Geometry check sheet. Reference: the model listing, model coordinates, mm. A direction names the side the tool comes from. Give positions to 0.01 mm unless a question says otherwise; leave off trailing zeros. Loops run counter-clockwise (first coordinate to the right, second up) from the corner with the lowest first, then second, coordinate; pieces in that order, holes last. Notation, with made-up numbers: (-30.5, 66.25) -> (15.5, 66.25) arc R27 cw to (15.5, 90.25) -> close; hole circle Ø5 at (55, 80). An arc over 180 degrees is marked (long way). Write item = value, one per line.
```python
from build123d import *

# Parameters (mm, degrees)
F0_W     = 12.7
F0_H     = 12.3
F1_DEPTH = 6.35
F2_W     = 6.35
F2_H     = 12.3
F3_DEPTH = 20.32
F4_R     = 1.9939
F5_DEPTH = 12.701
F7_DEPTH = 12.301
F9_DEPTH = 12.701


with BuildPart() as f1:
    # F0 (on Top) → F1 (new body)
    with BuildSketch(Plane.XY):
        Rectangle(F0_W, F0_H)
    extrude(amount=F1_DEPTH)

    # F2 (on face) → F3 (join)
    with BuildSketch(Plane.XY.offset(6.35)):
        with Locations((-3.175, 0)):
            Rectangle(F2_W, F2_H)
    extrude(amount=F3_DEPTH)

    # F4 (on face) → F5 (cut, through all)
    with BuildSketch(Plane.YZ.offset(6.35)):
        with Locations((0, 3.175)):
            Circle(F4_R)
    extrude(amount=-F5_DEPTH, mode=Mode.SUBTRACT)

    # F6 (on face) → F7 (cut, through all)
    with BuildSketch(Plane.XZ.offset(6.15)):
        Polygon((0, 20.955), (0, 23.495), (-2.54, 22.225), align=None)
    extrude(amount=-F7_DEPTH, mode=Mode.SUBTRACT)

    # F8 (on face) → F9 (cut, through all)
    with BuildSketch(Plane.YZ.offset(6.35)):
        with BuildLine():
            Line((-6.15, 5.08), (-6.15, 3.557324))
            ThreePointArc((-6.15, 3.557324), (-5.41976, 4.318662), (-6.15, 5.08))
        make_face()
        with BuildLine():
            Line((-6.15, 2.54), (-6.15, 1.017324))
            ThreePointArc((-6.15, 1.017324), (-5.41976, 1.778662), (-6.15, 2.54))
        make_face()
        with BuildLine():
            ThreePointArc((6.15, 2.54), (5.41976, 1.778662), (6.15, 1.017324))
            Line((6.15, 1.017324), (6.15, 2.54))
        make_face()
        with BuildLine():
            ThreePointArc((6.15, 5.08), (5.41976, 4.318662), (6.15, 3.557324))
            Line((6.15, 3.557324), (6.15, 5.08))
        make_face()
    extrude(amount=-F9_DEPTH, mode=Mode.SUBTRACT)


solid = f1.part
```
Item 1: Draft check along Z on faces 4 (the flat face through (3, 0, 6.35)), 5 (the flat face through (-1.25, -0.09, 22.87)), 6 (the cylindrical face through (0.09, 5.42, 1.79)), 7 (the flat face through (6.35, 0, 1)). Enter one of: +Z half, -Z half, draft (parallel to the pull), parting line (faces both ways), or undercut.
Answer:
face_4 = +Z half
face_5 = undercut
face_6 = undercut
face_7 = draft
Item 2: Tool access check on faces 1 (the cylindrical face through (0.09, -5.42, 1.76)), 2 (the flat face through (-1.29, -0.09, 21.6)), 3 (the flat face through (0, 0, 14)). Record the directions out of +Z, -Z, +X, -X, +Y, -Y that give a thin tool (end or side, any length) a straight path to the whole face; none if there is none.
Answer:
face_1 = +X, -X, -Y
face_2 = +X, +Y, -Y
face_3 = +Z, +X, +Y, -Y
Item 3: Section check C-C, the plane x = -4. Record the cut outline in (y, z) (3 decimals), plus the area to 3 significant figures.
Answer:
outline = (-6.15, 0) -> (6.15, 0) -> (6.15, 1.017) arc R0.762 cw to (6.15, 2.54) -> (6.15, 3.557) arc R0.762 cw to (6.15, 5.08) -> (6.15, 26.67) -> (-6.15, 26.67) -> (-6.15, 5.08) arc R0.762 cw to (-6.15, 3.557) -> (-6.15, 2.54) arc R0.762 cw to (-6.15, 1.017) -> close; hole circle Ø3.988 at (0, 3.175)
area = 312 mm^2
Item 4: Thickness scan on L1, parallel to Z at x = 0.5, y = 0; L2, parallel to X at y = -1.5, z = 10.75; L3, parallel to Z at x = 3, y = -5.25. Record the ranges inside material, lowest first. Write a range as [from, to].
Answer:
L1 = [0, 1.18], [5.17, 6.35]
L2 = [-6.35, 0]
L3 = [0, 6.35]
Item 5: Gauge pin test, flat ends, axial feed: pin 1 (3.5 mm diameter, centred on y = -1, z = 25.5, fed in from +X); pin 2 (2.5 mm diameter, centred on y = 0, z = 3.175, fed in from -X); pin 3 (7 mm diameter, centred on x = 4.5, y = 3, fed in from +Z). Record the tip position at first contact, or that the pin passes through.
Answer:
pin_1 = 0
pin_2 = through
pin_3 = 6.35
Item 6: Section check A-A, the plane y = 0. Record the cut outline in (x, z) (3 decimals), plus the area to 3 significant figures.
Answer:
outline = (-6.35, 0) -> (6.35, 0) -> (6.35, 1.181) -> (-6.35, 1.181) -> close; (-6.35, 5.169) -> (6.35, 5.169) -> (6.35, 6.35) -> (0, 6.35) -> (0, 20.955) -> (-2.54, 22.225) -> (0, 23.495) -> (0, 26.67) -> (-6.35, 26.67) -> close
area = 156 mm^2
Item 7: Section check B-B, the plane z = 4.25. Record the cut outline in (x, y), plus the area to 3 significant figures.
Answer:
outline = (-6.35, -5.42) -> (6.35, -5.42) -> (6.35, -1.68) -> (-6.35, -1.68) -> close; (-6.35, 1.68) -> (6.35, 1.68) -> (6.35, 5.42) -> (-6.35, 5.42) -> close
area = 95.1 mm^2
Item 8: Section check D-D, the plane y = -4.75. Record the cut outline in (x, z) (3 decimals).
Answer:
outline = (-6.35, 0) -> (6.35, 0) -> (6.35, 6.35) -> (0, 6.35) -> (0, 20.955) -> (-2.54, 22.225) -> (0, 23.495) -> (0, 26.67) -> (-6.35, 26.67) -> close
